Geometry: see drawing. Coordinates: mm, zero at the bounding-box minimum. Coordinates: 2 decimals unless noted, no trailing zeros. Write each loop counter-clockwise with the first axis right and the second up, starting at its lowest first coordinate (ties: lowest second). Pieces come first, ordered by that corner, then holes.
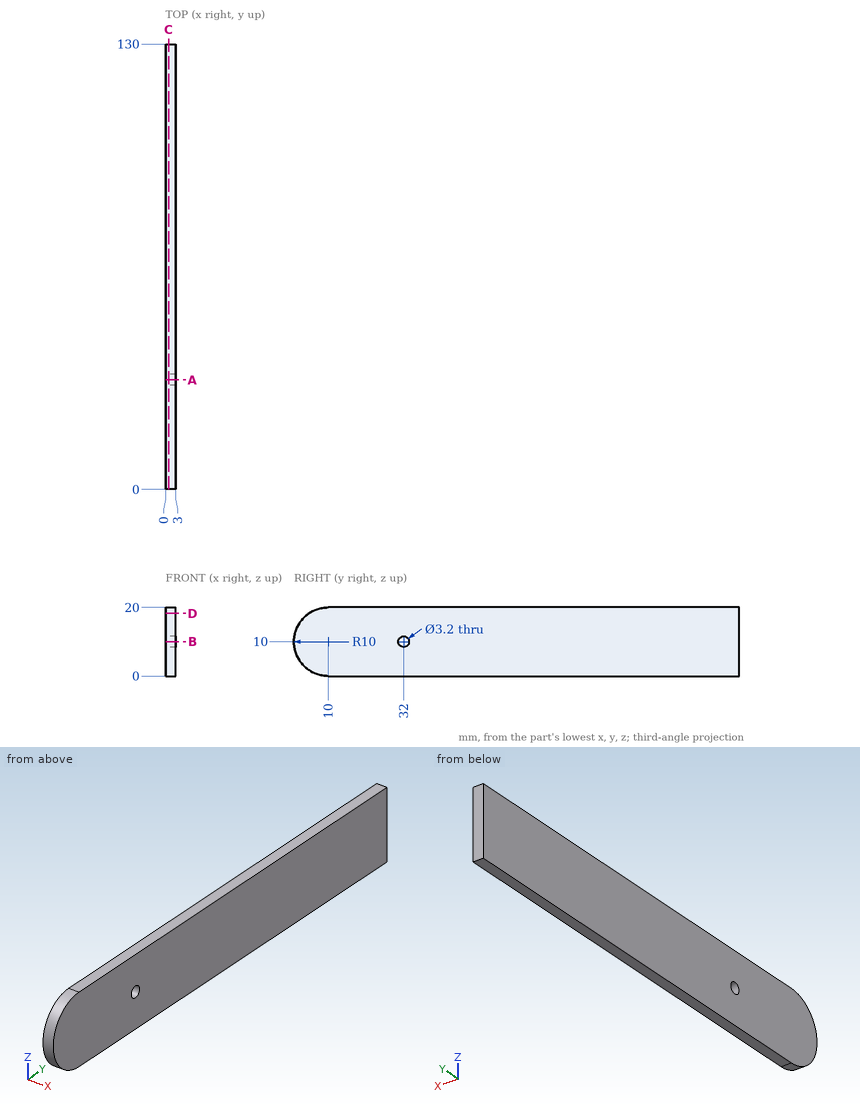
Item 1: Section D-D, the plane z = 18.25. Output: boundary loops of the cut face in (x, y), plus the area to 3 significant figures.
Derived:
outline: (0, 4.35) - (3, 4.35) - (3, 130) - (0, 130) - close
area: 377 mm2
Item 2: Pin query (flat end, axial travel): pin 1 (1.9 mm diameter, centred on y = 32, z = 10, fed in from +X). Return the tip coordinate at first contact, or that it passes through.
Derived:
pin 1: passes through
Item 3: Section A-A, the plane y = 32. Output: boundary loops of the cut face in (x, z), plus the area to 3 significant figures.
Derived:
outline: (0, 0) - (3, 0) - (3, 8.4) - (0, 8.4) - close; (0, 11.6) - (3, 11.6) - (3, 20) - (0, 20) - close
area: 50.4 mm2
Item 4: Section C-C, the plane x = 0.85. Output: boundary loops of the cut face in (y, z).
Derived:
outline: (10, 0) - (130, 0) - (130, 20) - (10, 20) arc R10 ccw to start; hole circle Ø3.2 at (32, 10)
Item 5: Material intervals for probe 1 along Z at (x, y) = (1.5, 32); probe 2 along Y at (x, z) = (1.15, 10); probe 3 along Y at (x, z) = (2.4, 9.5), sorted ascending.
Derived:
probe 1: z = 0 to 8.4, 11.6 to 20
probe 2: y = 0 to 30.4, 33.6 to 130
probe 3: y = 0.01 to 30.48, 33.52 to 130
Item 6: Section B-B, the plane z = 10. Output: boundary loops of the cut face in (x, y), plus the area to 3 significant figures.
Derived:
outline: (0, 0) - (3, 0) - (3, 30.4) - (0, 30.4) - close; (0, 33.6) - (3, 33.6) - (3, 130) - (0, 130) - close
area: 380 mm2
